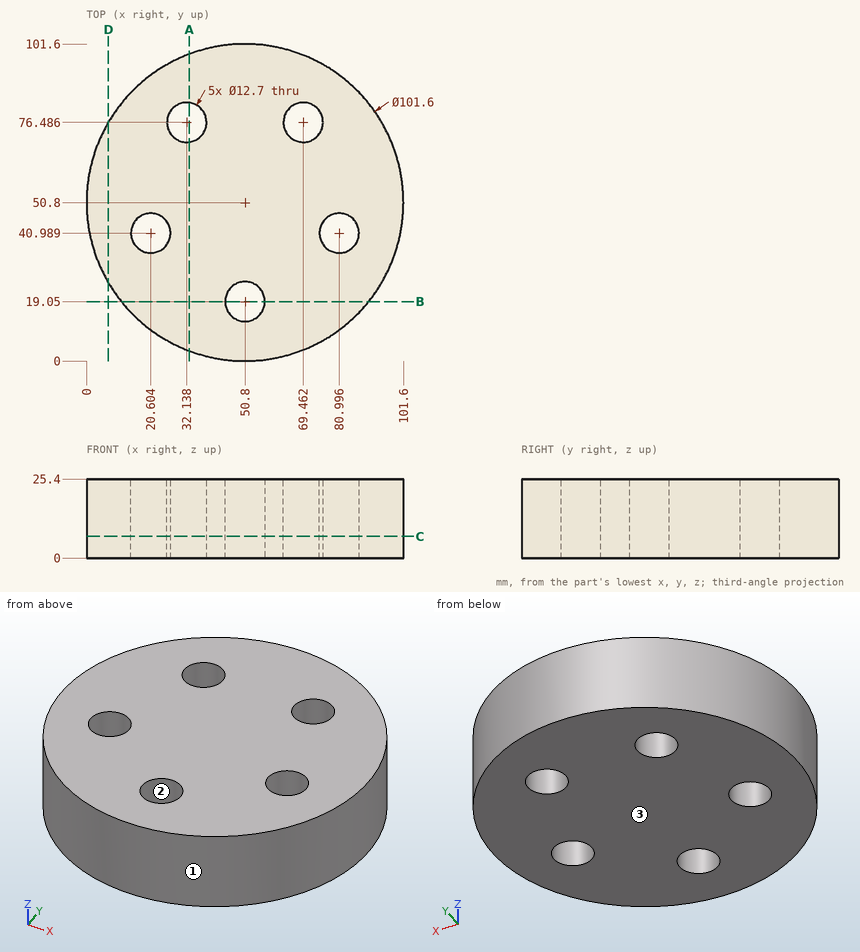
Geometry: see drawing. Coordinates: mm, zero at the bounding-box minimum. Round coordinates to 2 decimals unless told otherwise and drop trailing zeros. Write each loop counter-clockwise with the first axis right and the second up, starting at its lowest first coordinate (ties: lowest second). Pieces come first, ordered by that corner, then holes. Notation, with made-up numbers: M 38,-25.5 L 44,-25.5 A14 cw 44,-2.5 Z; hole C 6.25,43 d4. An arc over 180 degrees is marked long. Answer as a JSON object with one key per item and string values. Group by question number.
(1) Mould query, pull axis Y, two halves, no side actions, for the marked faces 1, 2 and 3. Classes: +Y half, -Y half, draft (parallel to the pull), parting line (faces both ways), or undercut.
(2) Section query D-D on x = 7. Output: boundary loops of the cut face in (y, z), then the cut area to 3 significant figures.
(3) Section query C-C on z = 7. State how many separate pieces and enclosed holes the cut face has, then the cut area to 3 significant figures.
(4) Section query A-A on x = 33. Output: boundary loops of the cut face in (y, z) (1 decimal), then the cut area to 3 significant figures.
(5) Ray query, line 1 (X direction, y = 79, z = 11.25) (1 decimal); line 2 (X direction, y = 73, z = 18.5) (1 decimal); line 3 (Y direction, x = 50.5, z = 7.25). Return the intervals inside material, ascending. Write a range as [from, to].
(6) Section query B-B on y = 19.05. Output: boundary loops of the cut face in (x, z).
(7) First-contact query: pin 1 (12 mm diameter, centred on y = 80, z = 13, fed in from -X); pin 2 (1.5 mm diameter, centred on x = 52.5, z = 15, fed in from -Y); pin 3 (4 mm diameter, centred on x = 30, z = 7.5, fed in from +Y); pin 4 (16.5 mm diameter, centred on x = 50.8, y = 19.05, fed in from +Z). Flat tips, straight axial feed; report the tip coordinate or a pass-through.
Computed values:
{
 "1": {"face 1": "parting line", "face 2": "undercut", "face 3": "draft"},
 "2": {"outline": "M 25.07,0 L 76.53,0 L 76.53,25.4 L 25.07,25.4 Z", "area": "1,310 mm^2"},
 "3": {"separate pieces": "1", "enclosed holes": "5", "area": "7,470 mm^2"},
 "4": {"outline": "M 3.2,0 L 70.2,0 L 70.2,25.4 L 3.2,25.4 Z; M 82.8,0 L 98.4,0 L 98.4,25.4 L 82.8,25.4 Z", "area": "2,100 mm^2"},
 "5": {"line 1": "[8.5, 26.3], [38, 63.6], [75.3, 93.1]", "line 2": "[5.1, 26.8], [37.4, 64.2], [74.8, 96.5]", "line 3": "[0, 12.71], [25.39, 101.6]"},
 "6": {"outline": "M 11.14,0 L 44.45,0 L 44.45,25.4 L 11.14,25.4 Z; M 57.15,0 L 90.46,0 L 90.46,25.4 L 57.15,25.4 Z"},
 "7": {"pin 1": "x = 5.61", "pin 2": "y = 0.01", "pin 3": "y = 97.99", "pin 4": "z = 25.4"}
}
